```python
from build123d import *

# Parameters (mm, degrees)
SKETCH1_W                = 75
SKETCH1_H                = 19
BOSS_EXTRUDE1_DEPTH      = 10
SKETCH4_W                = 16
SKETCH4_H                = 19
CUT_EXTRUDE1_DEPTH       = 5
BOSS_EXTRUDE2_DEPTH      = 45.5
BOSS_EXTRUDE2_DEPTH_BACK = 29.5
SKETCH6_W                = 26.5
SKETCH6_H                = 19
CUT_EXTRUDE2_DEPTH       = 2


with BuildPart() as part:
    # Sketch1 → Boss-Extrude1 (new body)
    with BuildSketch(Plane(origin=(0, 0, 0), x_dir=(1, 0, 0), z_dir=(0, 1, 0))):
        Rectangle(SKETCH1_W, SKETCH1_H)
    extrude(amount=-BOSS_EXTRUDE1_DEPTH)

    # Sketch4 → Cut-Extrude1 (cut)
    with BuildSketch(Plane(origin=(0, 0, 0), x_dir=(1, 0, 0), z_dir=(0, 1, 0))):
        Rectangle(SKETCH4_W, SKETCH4_H)
    extrude(amount=-CUT_EXTRUDE1_DEPTH, mode=Mode.SUBTRACT)

    # Sketch5 → Boss-Extrude2 (add, two sides: drawn at the far end of the back side and taken through both)
    with BuildSketch(Plane.ZY.offset(-8).offset(-BOSS_EXTRUDE2_DEPTH_BACK)):
        Polygon((-2.5, -5), (0, 2), (2.5, -5), align=None)
    extrude(amount=BOSS_EXTRUDE2_DEPTH + BOSS_EXTRUDE2_DEPTH_BACK)

    # Sketch6 → Cut-Extrude2 (cut)
    with BuildSketch(Plane(origin=(0, 0, 0), x_dir=(1, 0, 0), z_dir=(0, 1, 0))):
        with Locations((-21.25, 0)):
            Rectangle(SKETCH6_W, SKETCH6_H)
        with Locations((21.25, 0)):
            Rectangle(SKETCH6_W, SKETCH6_H)
    extrude(amount=CUT_EXTRUDE2_DEPTH, mode=Mode.SUBTRACT)


solid = part.part
```
Read the model definition and answer for the solid it produces. Units are mm, in the model's axes. A direction names the side the tool comes from. Give positions to 0.01 mm unless a question says otherwise; leave off trailing zeros. Write each loop counter-clockwise with the first axis right and the second up, starting at its lowest first coordinate (ties: lowest second). Pieces come first, ordered by that corner, then holes. Notation, with made-up numbers: (57.25, 2) - (96.25, 2) arc R17 cw to (96.25, 21) - close; hole circle Ø5 at (76.25, -38). An arc over 180 degrees is marked (long way). Write item = value, one per line. Start each with the question number.
Item 1: Each of these flat-tipped pins is pushed along its axis until it touches: P1, Ø2, axis at x = -3.5, z = 4.5, coming from the +Y side; P2, Ø5.5, axis at x = -26.5, z = 3.5, coming from the +Y side. Where does it stop, or does it pass through?
Item 2: Find section D-D (x = 16). Give the vertices of the cut face in (y, z).
Item 3: A tool of negligible diameter and unlimited length cuts with its end or side. For faces 4 (the flat face through (0.112, -1.549, -1.268)), 5 (the flat face through (34.5, 1, 0)), 6 (the flat face through (0, -5, 6)), from which of +Z, -Z, +X, -X, +Y, -Y can it reach the whole face along a straight path? Write none if from no direction.
Item 4: Find section B-B (x = 3.5). Give the vertices of the cut face in (y, z), then the cut area to 4 significant figures.
Item 5: The mould has two halves that part along X. Classify faces 1 (the flat face through (8, 1, 0)), 2 (the flat face through (-1, -6, 9.5)), 3 (the flat face through (-37.5, -5, 0)): +X half, -X half, draft (parallel to the pull), parting line (faces both ways), or undercut.
Item 6: Find the intervals of material crossed by probe 1 along X at (y, z) = (-1.75, -6.25); probe 2 along Y at (x, z) = (-15.5, -2); probe 3 along Y at (x, z) = (7, -7.75), in increasing order. Write a range as [from, to].
Item 7: Find section A-A (z = -3.25). Give the vertices of the cut face in (x, y), then the cut area to 3 significant figures.
Item 8: Find section C-C (y = -3.75). Give the vertices of the cut face in (x, z).
Response:
q1.P1 = -5
q1.P2 = 0
q2.outline = (-10, -9.5) - (0, -9.5) - (0, 9.5) - (-10, 9.5) - close
q3.face_4 = -Z, +Y
q3.face_5 = +Z, -Z, +Y
q3.face_6 = +Z, +Y
q4.outline = (-10, -9.5) - (-5, -9.5) - (-5, -2.5) - (2, 0) - (-5, 2.5) - (-5, 9.5) - (-10, 9.5) - close
q4.area = 112.5 mm²
q5.face_1 = undercut
q5.face_2 = draft
q5.face_3 = -X half
q6.probe_1 = [-37.5, -8], [8, 37.5]
q6.probe_2 = [-10, 0]
q6.probe_3 = [-10, -5]
q7.outline = (-37.5, -10) - (37.5, -10) - (37.5, 0) - (8, 0) - (8, -5) - (-8, -5) - (-8, 0) - (-37.5, 0) - close
q7.area = 670 mm²
q8.outline = (-37.5, -9.5) - (-8, -9.5) - (-8, -2.05) - (8, -2.05) - (8, -9.5) - (37.5, -9.5) - (37.5, 9.5) - (8, 9.5) - (8, 2.05) - (-8, 2.05) - (-8, 9.5) - (-37.5, 9.5) - close
